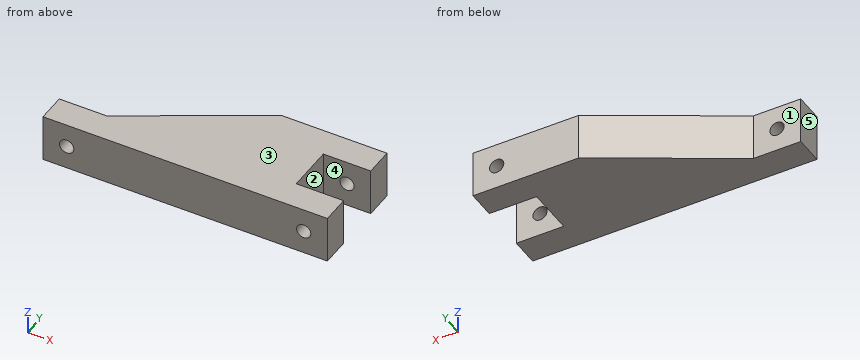
```python
from build123d import *

# Parameters (mm, degrees)
BOSS_EXTRUDE1_DEPTH     = 50
SKETCH2_R               = 7.5
CUT_EXTRUDE1_DEPTH      = 81
CUT_EXTRUDE1_DEPTH_BACK = 31


with BuildPart() as part:
    # Sketch1 → Boss-Extrude1 (new body)
    with BuildSketch(Plane.XY):
        Polygon((-300, 0), (0, 0), (0, 30), (-50, 30), (-50, 80), (0, 80), (0, 110), (-111.435935394, 110), (-250, 30), (-300, 30), align=None)
    extrude(amount=BOSS_EXTRUDE1_DEPTH)

    # Sketch2 → Cut-Extrude1 (cut, two sides)
    with BuildSketch(Plane(origin=(0, 30, 0), x_dir=(1, 0, 0), z_dir=(0, 1, 0))) as cut_extrude1_sk:
        with Locations((-275, -25)):
            Circle(SKETCH2_R)
        with Locations((-25, -25)):
            Circle(SKETCH2_R)
    extrude(amount=CUT_EXTRUDE1_DEPTH, mode=Mode.SUBTRACT)
    extrude(cut_extrude1_sk.sketch, amount=-CUT_EXTRUDE1_DEPTH_BACK, mode=Mode.SUBTRACT)


solid = part.part
```
Could you check a few things on this model? Use its own coordinates, in mm. Face numbers are marked on the shaded views. A direction names the side the tool comes from. Round coordinates to 2 decimals unless told otherwise and drop trailing zeros. Order: outer loops, then holes, each group sorted by start corner. A loop starts at its lowest first (then second) coordinate and runs counter-clockwise, first axis right, second up. Notation, with made-up numbers: (66.25, 30.5) -> (77.25, 30.5) arc R26 ccw to (77.25, 44.5) -> close; hole circle Ø7 at (-27, 70). An arc over 180 degrees is marked (long way). One line per question, with ' | ' between items.
Q1. If we section it at A-A on x = -275: Write out the boundary of the cut face in (y, z).
Computed values:
outline: (0, 0) -> (30, 0) -> (30, 17.5) -> (0, 17.5) -> close; (0, 32.5) -> (30, 32.5) -> (30, 50) -> (0, 50) -> close
Q2. If we section it at C-C on x = -25: Write out the boundary of the cut face in (y, z), plus the area to 3 significant figures.
Computed values:
outline: (0, 0) -> (30, 0) -> (30, 17.5) -> (0, 17.5) -> close; (0, 32.5) -> (30, 32.5) -> (30, 50) -> (0, 50) -> close; (80, 0) -> (110, 0) -> (110, 17.5) -> (80, 17.5) -> close; (80, 32.5) -> (110, 32.5) -> (110, 50) -> (80, 50) -> close | area: 2,100 mm²
Q3. If I drill on line 1 (X direction, y = 16, z = 25); line 2 (Z direction, x = -25, y = 98.25); line 3 (X direction, y = 20, z = 21), over which ranges is the centre line in solid material (lowest first)? Write a range as from..to.
Computed values:
line 1: -300..-282.5, -267.5..-32.5, -17.5..0 | line 2: 0..17.5, 32.5..50 | line 3: -300..-281.34, -268.66..-31.34, -18.66..0
Q4. If we section it at B-B on z = 25: Write out the boundary of the cut face in (x, y), plus the area to 3 significant figures.
Computed values:
outline: (-300, 0) -> (-282.5, 0) -> (-282.5, 30) -> (-300, 30) -> close; (-267.5, 0) -> (-32.5, 0) -> (-32.5, 30) -> (-50, 30) -> (-50, 80) -> (-32.5, 80) -> (-32.5, 110) -> (-111.44, 110) -> (-250, 30) -> (-267.5, 30) -> close; (-17.5, 0) -> (0, 0) -> (0, 30) -> (-17.5, 30) -> close; (-17.5, 80) -> (0, 80) -> (0, 110) -> (-17.5, 110) -> close | area: 19,600 mm²
Q5. If we section it at D-D on z = 40: Write out the boundary of the cut face in (x, y).
Computed values:
outline: (-300, 0) -> (0, 0) -> (0, 30) -> (-50, 30) -> (-50, 80) -> (0, 80) -> (0, 110) -> (-111.44, 110) -> (-250, 30) -> (-300, 30) -> close
Q6. Which directions (+Z, -Z, +X, -X, +Y, -Y) give clear straight access to the entire face, cutting with the end or side of a thin tool? Please do the marked faces 4 and 5.
Computed values:
face 4: +Z, -Z, +X | face 5: +Z, -Z, -X, +Y, -Y
Q7. We'd pull the mould along Y, two halves only. Please class the marked faces 1, 2 and 3: released by +Y, released by -Y, zero draft, split by the parting line, or undercut.
Computed values:
face 1: released by +Y | face 2: undercut | face 3: zero draft
Q8. I'm going to push flat-ended pins straight in: pin 1 (3 mm diameter, centred on y = 61, z = 26, fed in from -X); pin 2 (6 mm diameter, centred on x = -216, z = 35.5, fed in from +Y); pin 3 (2 mm diameter, centred on y = 47.5, z = 21.5, fed in from -X). Where does each tip first touch, or does it pass through?
Computed values:
pin 1: x = -198.9 | pin 2: y = 51.36 | pin 3: x = -221.42
